from build123d import *

# Parameters (mm, degrees)
F0_R     = 15.875
F1_DEPTH = 15.875
F2_R     = 4.445
F3_DEPTH = 44.45
F4_R     = 4.445
F5_DEPTH = 76.2


with BuildPart() as f1:
    # F0 (on Right) → F1 (new body, symmetric)
    with BuildSketch(Plane.YZ):
        Circle(F0_R)
    extrude(amount=F1_DEPTH, both=True)

    # F2 (on face) → F3 (join)
    with BuildSketch(Plane.YZ.offset(15.875)):
        Circle(F2_R)
    extrude(amount=F3_DEPTH)

    # F4 (on Front) → F5 (join, symmetric)
    with BuildSketch(Plane.XZ):
        Circle(F4_R)
    extrude(amount=F5_DEPTH, both=True)

    # F6 (on Top) → F7 (revolve)
    with BuildSketch(Plane.XY):
        with BuildLine():
            Line((-4.445, 76.2), (4.445, 76.2))
            Line((4.445, 76.2), (10.16, 76.2))
            ThreePointArc((10.16, 76.2), (0, 86.36), (-10.16, 76.2))
            Line((-10.16, 76.2), (-4.445, 76.2))
        make_face()
    revolve(axis=Axis((14.6032162011, 76.2, 0), (1, 0, 0)))

    # F8 (on Top) → F9 (revolve)
    with BuildSketch(Plane.XY):
        with BuildLine():
            Line((10.16, -76.2), (-10.16, -76.2))
            ThreePointArc((-10.16, -76.2), (0, -86.36), (10.16, -76.2))
        make_face()
    revolve(axis=Axis((4.1940081865, -76.2, 0), (1, 0, 0)))


solid = f1.part
Model file for the job. Use its own axes, mm. A direction names the side the tool comes from. Round coordinates to 2 decimals unless told otherwise and drop trailing zeros. Order: outer loops, then holes, each group sorted by start corner. A loop starts at its lowest first (then second) coordinate and runs counter-clockwise, first axis right, second up.
(1) Pin check, flat tips, straight feed: pin 1 (8 mm diameter, centred on y = -24, z = 2, fed in from -X) (3 decimals); pin 2 (1 mm diameter, centred on y = -57.5, z = 4.5, fed in from +X); pin 3 (8 mm diameter, centred on x = 17.5, z = 6.5, fed in from +Y). Stop position of each tip, or through.
(2) Drill centre lines: line 1 (X direction, y = -5.5, z = -7) (3 decimals); line 2 (Z direction, x = 21, y = -0.5); line 3 (Y direction, x = -3.5, z = 6). Where is each one in solid material? Low to high.
(3) Band-saw the part on C-C (y = 0). List the corners of the cut face in (x, z) (3 decimals), then the cut area to 3 significant figures.
(4) Band-saw the part on B-B (z = 0). List the corners of the cut face in (x, y) (3 decimals).
(5) Band-saw the part on A-A (x = 0). List the corners of the cut face in (y, z) (3 decimals).
(6) Pull direction Y, two halves, no side cores. Call faces 1 (the face through (37.79, -0.96, -4.34)), 2 (the face through (-0.96, 40.79, -4.34)), 3 (the face through (-15.875, 0, 0)): released by +Y, released by -Y, zero draft, split by the parting line, or undercut.
(7) 3-axis set-ups, long thin cutter, end or side, ignore diameter. For faces 4 (the face through (15.875, 3.3, -3.3)), 5 (the face through (-0.96, -41.51, -4.34)), 6 (the face through (60.325, 0, 0)): which of +Z, -Z, +X, -X, +Y, -Y reach the whole face in a straight line?
(8) Band-saw the part on D-D (y = 47). List the corners of the cut face in (x, z) (3 decimals), then the cut area to 3 significant figures.
Verdict:
1. pin 1: stops at x = -4.445
1. pin 2: stops at x = 1.94
1. pin 3: stops at y = 15.62
2. line 1: x = -15.875 to 15.875
2. line 2: z = -4.42 to 4.42
2. line 3: y = -83.61 to -68.79, -14.7 to 14.7, 68.79 to 83.61
3. outline: (-15.875, -15.875) - (15.875, -15.875) - (15.875, -4.445) - (60.325, -4.445) - (60.325, 4.445) - (15.875, 4.445) - (15.875, 15.875) - (-15.875, 15.875) - close
3. area: 1,400 mm2
4. outline: (-15.875, -15.875) - (-4.445, -15.875) - (-4.445, -67.064) arc R10.16 ccw (long way) to (4.445, -67.064) - (4.445, -15.875) - (15.875, -15.875) - (15.875, -4.445) - (60.325, -4.445) - (60.325, 4.445) - (15.875, 4.445) - (15.875, 15.875) - (4.445, 15.875) - (4.445, 67.064) arc R10.16 ccw (long way) to (-4.445, 67.064) - (-4.445, 15.875) - (-15.875, 15.875) - close
5. outline: (-67.064, -4.445) - (-15.24, -4.445) arc R15.875 ccw to (15.24, -4.445) - (67.064, -4.445) arc R10.16 ccw (long way) to (67.064, 4.445) - (15.24, 4.445) arc R15.875 ccw to (-15.24, 4.445) - (-67.064, 4.445) arc R10.16 ccw (long way) to start
6. face 1: split by the parting line
6. face 2: undercut
6. face 3: zero draft
7. face 4: +X
7. face 5: none
7. face 6: +Z, -Z, +X, +Y, -Y
8. outline: circle Ø8.89 at (0, 0)
8. area: 62.1 mm2
